```python
from build123d import *

# Parameters (mm, degrees)
F0_R     = 14.2875
F1_DEPTH = 25.4
F2_DEPTH = 35.306
F3_R     = 5.08


with BuildPart() as f1:
    # F0 (on Front) → F1 (new body)
    with BuildSketch(Plane.XZ):
        with BuildLine():
            Line((9.780704698, 26.8489932886), (0, 28.575))
            ThreePointArc((0, 28.575), (-28.575, 0), (0, -28.575))
            Line((0, -28.575), (9.7850073358, -26.8474255086))
            ThreePointArc((9.7850073358, -26.8474255086), (23.4108651017, -16.3848106547), (28.575, 0))
            ThreePointArc((28.575, 0), (23.4095521288, 16.3866864902), (9.780704698, 26.8489932886))
        make_face()
        with BuildLine():
            ThreePointArc((-13.4703841816, 4.7625), (0, 14.2875), (13.4703841816, 4.7625))
            Line((13.4703841816, 4.7625), (19.05, 4.7625))
            Line((19.05, 4.7625), (19.05, -4.7625))
            Line((19.05, -4.7625), (13.4703841816, -4.7625))
            ThreePointArc((13.4703841816, -4.7625), (0, -14.2875), (-13.4703841816, -4.7625))
            Line((-13.4703841816, -4.7625), (-19.05, -4.7625))
            Line((-19.05, -4.7625), (-19.05, 4.7625))
            Line((-19.05, 4.7625), (-13.4703841816, 4.7625))
        make_face(mode=Mode.SUBTRACT)
        with BuildLine():
            Line((53.975, 19.05), (9.780704698, 26.8489932886))
            ThreePointArc((9.780704698, 26.8489932886), (23.4095521288, 16.3866864902), (28.575, 0))
            ThreePointArc((28.575, 0), (23.4108651017, -16.3848106547), (9.7850073358, -26.8474255086))
            Line((9.7850073358, -26.8474255086), (53.949834283, -19.0499833776))
            ThreePointArc((53.949834283, -19.0499833776), (34.9250041556, 0.0125828612), (53.975, 19.05))
        make_face()
        with BuildLine():
            ThreePointArc((73.025, 0), (67.4453841816, 13.4703841816), (53.975, 19.05))
            ThreePointArc((53.975, 19.05), (34.9250041556, 0.0125828612), (53.949834283, -19.0499833776))
            ThreePointArc((53.949834283, -19.0499833776), (67.4364838166, -13.4792786697), (73.025, 0))
        make_face()
        with Locations((53.975, 0)):
            Circle(F0_R, mode=Mode.SUBTRACT)
        with BuildLine():
            ThreePointArc((-13.4703841816, -4.7625), (-14.2875, 0), (-13.4703841816, 4.7625))
            Line((-13.4703841816, 4.7625), (-19.05, 4.7625))
            Line((-19.05, 4.7625), (-19.05, -4.7625))
            Line((-19.05, -4.7625), (-13.4703841816, -4.7625))
        make_face()
    extrude(amount=F1_DEPTH)

    # F0 (on Front) → F2 (join)
    with BuildSketch(Plane.XZ):
        with BuildLine():
            Line((9.780704698, 26.8489932886), (0, 28.575))
            ThreePointArc((0, 28.575), (-28.575, 0), (0, -28.575))
            Line((0, -28.575), (9.7850073358, -26.8474255086))
            ThreePointArc((9.7850073358, -26.8474255086), (23.4108651017, -16.3848106547), (28.575, 0))
            ThreePointArc((28.575, 0), (23.4095521288, 16.3866864902), (9.780704698, 26.8489932886))
        make_face()
        with BuildLine():
            ThreePointArc((-13.4703841816, 4.7625), (0, 14.2875), (13.4703841816, 4.7625))
            Line((13.4703841816, 4.7625), (19.05, 4.7625))
            Line((19.05, 4.7625), (19.05, -4.7625))
            Line((19.05, -4.7625), (13.4703841816, -4.7625))
            ThreePointArc((13.4703841816, -4.7625), (0, -14.2875), (-13.4703841816, -4.7625))
            Line((-13.4703841816, -4.7625), (-19.05, -4.7625))
            Line((-19.05, -4.7625), (-19.05, 4.7625))
            Line((-19.05, 4.7625), (-13.4703841816, 4.7625))
        make_face(mode=Mode.SUBTRACT)
        with BuildLine():
            ThreePointArc((-13.4703841816, -4.7625), (-14.2875, 0), (-13.4703841816, 4.7625))
            Line((-13.4703841816, 4.7625), (-19.05, 4.7625))
            Line((-19.05, 4.7625), (-19.05, -4.7625))
            Line((-19.05, -4.7625), (-13.4703841816, -4.7625))
        make_face()
    extrude(amount=-F2_DEPTH)

    # F3
    f3_edges = [f1.edges().sort_by_distance(p)[0] for p in [
        (13.470384, 4.953, -4.7625),
        (13.470384, 4.953, 4.7625),
    ]]
    fillet(f3_edges, radius=F3_R)


solid = f1.part
```
Design review of the part built by this model. Coordinates are the model's own, in mm. A direction names the side the tool comes from. Give positions to 0.01 mm unless a question says otherwise; leave off trailing zeros. Order: outer loops, then holes, each group sorted by start corner. A loop starts at its lowest first (then second) coordinate and runs counter-clockwise, first axis right, second up. Notation, with made-up numbers: (72, -9) - (121, -9) arc R16 cw to (121, 14) - close; hole circle Ø9 at (2.25, 78). An arc over 180 degrees is marked (long way). Use a Markdown table: item, result. Add a question column.
(1) Add section C-C on x = 62. Give the boundary of the cut face in (y, z).
(2) Add section B-B on z = 6. Give the boundary of the cut face in (x, y), then the cut area to 3 significant figures.
(3) Clearance check with flat-ended pins moving along their axes: P1, Ø6, axis at x = 50, z = -20.5, coming from the -Y side; P2, Ø1, axis at y = -12.5, z = 4, coming from the +X side; P3, Ø8, axis at x = 4, z = 5.5, coming from the -Y side; P4, Ø1.9, axis at x = 17.5, y = -4, coming from the -Z side. State where each tip first meets the part, or that it passes through.
(4) Mouldability with a two-part tool opening along Z and no side actions: class faces 1 (the face through (73.02, -12.52, -0.43)), 2 (the face through (18, 5, 4.762)), 3 (the face through (39, 0, 2)) as +Z half, -Z half, draft (parallel to the pull), parting line (faces both ways), or undercut.
(5) Machinability: for faces 4 (the face through (14.193, 4.528, 5.413)), 5 (the face through (-28.57, 4.53, 0.63)), which of the approach directions +Z, -Z, +X, -X, +Y, -Y give a long, thin tool a straight path to every point of the face, cutting with its end or side? Answer none if there is none.
(6) Add section A-A on y = -14. Give the number of separate pieces and of enclosed holes in the cut face, then the cut area to 3 significant figures.
(7) Wall thickness on probe 1 along X at (y, z) = (-14, -0.5); probe 2 along X at (y, z) = (-10.5, 13); probe 3 along Y at (x, z) = (29, -16.5): over which ranges is each line inside the solid? List them lowest first. Write a range as [from, to].
Report:
| question | item | result |
|---|---|---|
| 1 | outline | (-25.4, -17.28) - (0, -17.28) - (0, -11.82) - (-25.4, -11.82) - close; (-25.4, 11.82) - (0, 11.82) - (0, 17.28) - (-25.4, 17.28) - close |
| 2 | outline | (-27.94, -25.4) - (-12.97, -25.4) - (-12.97, 35.31) - (-27.94, 35.31) - close; (13.36, -25.4) - (41.01, -25.4) - (41.01, 0) - (27.94, 0) - (27.94, 35.31) - (13.36, 35.31) - close; (66.94, -25.4) - (72.06, -25.4) - (72.06, 0) - (66.94, 0) - close |
| 2 | area | 2,260 mm² |
| 3 | P1 | stops at y = -25.4 |
| 3 | P2 | stops at x = 72.7 |
| 3 | P3 | passes through |
| 3 | P4 | stops at z = -25.65 |
| 4 | face 1 | parting line |
| 4 | face 2 | undercut |
| 4 | face 3 | draft |
| 5 | face 4 | +Y, -Y |
| 5 | face 5 | -X, +Y, -Y |
| 6 | separate pieces | 1 |
| 6 | enclosed holes | 2 |
| 6 | area | 3,090 mm² |
| 7 | probe 1 | x = [-28.57, -14.28], [19.05, 39.7], [68.25, 73.02] |
| 7 | probe 2 | x = [-25.45, -5.93], [5.93, 48.05], [59.9, 67.9] |
| 7 | probe 3 | y = [-25.4, 0] |
